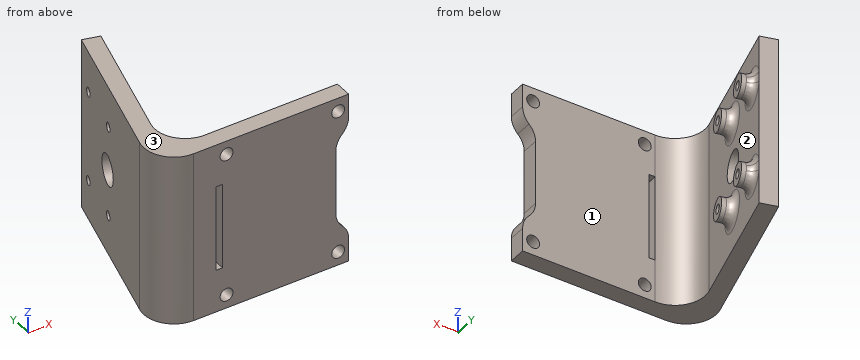
```python
from build123d import *
from build123d.topology import SkipClean

# Parameters (mm, degrees)
ESTRUSIONE_ESTRUSIONE1_DEPTH = 40
RACCORDO1_R                  = 7
SCHIZZO2_W                   = 1.5
SCHIZZO2_H                   = 20
TAGLIO_ESTRUSIONE1_DEPTH     = 40
SCHIZZO3_R                   = 1.05
SCHIZZO3_R_2                 = 3.5
TAGLIO_ESTRUSIONE2_DEPTH     = 40
SCHIZZO4_R                   = 2.5
SCHIZZO4_R_2                 = 1.05
ESTRUSIONE_ESTRUSIONE2_DEPTH = 3
RACCORDO2_R                  = 2
SCHIZZO5_R                   = 1.5
TAGLIO_ESTRUSIONE3_DEPTH     = 17
TAGLIO_ESTRUSIONE4_DEPTH     = 10
RACCORDO3_R                  = 5
RACCORDO4_R                  = 5


with BuildPart() as part:
    # Schizzo1 → Estrusione-Estrusione1 (new body)
    with BuildSketch(Plane.XY):
        Polygon((0, 0), (-40, 0), (-29.647238196, 38.637033052), (-33.510941501, 39.672309232), (-45.212901491, -4), (0, -4), align=None)
    extrude(amount=ESTRUSIONE_ESTRUSIONE1_DEPTH)

    # Raccordo1
    raccordo1_edges = [part.edges().sort_by_distance(p)[0] for p in [
        (-45.212901491, -4, 20),
        (-40, 0, 20),
    ]]
    fillet(raccordo1_edges, radius=RACCORDO1_R)

    # Schizzo2 → Taglio-Estrusione1 (cut)
    with BuildSketch(Plane(origin=(0, 0, 0), x_dir=(1, 0, 0), z_dir=(0, 1, 0))):
        with Locations((-30.12742239, -20)):
            Rectangle(SCHIZZO2_W, SCHIZZO2_H)
    extrude(amount=-TAGLIO_ESTRUSIONE1_DEPTH, mode=Mode.SUBTRACT)

    # Schizzo3 → Taglio-Estrusione2 (cut)
    with BuildSketch(Plane(origin=(-41.184211381, 11.03527618, 0), x_dir=(0, 0, 1), z_dir=(-0.9659258262890673, 0.2588190451025247, 0))):
        with Locations(Location((30.402866557, 25.309568218, 0), (0, 0, 270))):
            Circle(SCHIZZO3_R)
        with Locations(Location((9.20859967, 25.309568218, 0), (0, 0, 270))):
            Circle(SCHIZZO3_R)
        with Locations(Location((30.402866557, 13.009568218, 0), (0, 0, 270))):
            Circle(SCHIZZO3_R)
        with Locations(Location((9.20859967, 13.009568218, 0), (0, 0, 270))):
            Circle(SCHIZZO3_R)
        with Locations(Location((19.902866557, 13.409568216, 0), (0, 0, 270))):
            Circle(SCHIZZO3_R_2)
    extrude(amount=-TAGLIO_ESTRUSIONE2_DEPTH, mode=Mode.SUBTRACT)

    # Schizzo4 → Estrusione-Estrusione2 (add)
    # profile 1 of 4: a face of its own
    with SkipClean():  # the faces are left unmerged after this step: merging them gives an invalid solid
        with BuildSketch(Plane(origin=(-37.320508076, 10, 0), x_dir=(0, 0, -1), z_dir=(0.9659258262890674, -0.2588190451025245, 0))):
            with Locations(Location((-9.20859967, 13.009568218, 0), (0, 0, 270))):
                Circle(SCHIZZO4_R)
            with Locations(Location((-9.20859967, 13.009568218, 0), (0, 0, 90))):
                Circle(SCHIZZO4_R_2, mode=Mode.SUBTRACT)
        # profile 2 of 4: a face of its own
        with BuildSketch(Plane(origin=(-37.320508076, 10, 0), x_dir=(0, 0, -1), z_dir=(0.9659258262890674, -0.2588190451025245, 0))):
            with Locations(Location((-30.402866557, 13.009568218, 0), (0, 0, 270))):
                Circle(SCHIZZO4_R)
            with Locations(Location((-30.402866557, 13.009568218, 0), (0, 0, 270))):
                Circle(SCHIZZO4_R_2, mode=Mode.SUBTRACT)
        # profile 3 of 4: a face of its own
        with BuildSketch(Plane(origin=(-37.320508076, 10, 0), x_dir=(0, 0, -1), z_dir=(0.9659258262890674, -0.2588190451025245, 0))):
            with Locations(Location((-30.402866557, 25.309568218, 0), (0, 0, 270))):
                Circle(SCHIZZO4_R)
            with Locations(Location((-30.402866557, 25.309568218, 0), (0, 0, 270))):
                Circle(SCHIZZO4_R_2, mode=Mode.SUBTRACT)
        # profile 4 of 4: a face of its own
        with BuildSketch(Plane(origin=(-37.320508076, 10, 0), x_dir=(0, 0, -1), z_dir=(0.9659258262890674, -0.2588190451025245, 0))):
            with Locations(Location((-9.20859967, 25.309568218, 0), (0, 0, 270))):
                Circle(SCHIZZO4_R)
            with Locations(Location((-9.20859967, 25.309568218, 0), (0, 0, 90))):
                Circle(SCHIZZO4_R_2, mode=Mode.SUBTRACT)
        extrude(amount=ESTRUSIONE_ESTRUSIONE2_DEPTH)
    add(part.part.scale(1), mode=Mode.REPLACE)  # the faces are merged on a copy

    # Raccordo2
    raccordo2_edges = [part.edges().sort_by_distance(p)[0] for p in [
        (-30.122862185, 36.86198016, 9.20859967),
        (-33.306336439, 24.981092497, 9.20859967),
        (-33.306336439, 24.981092497, 30.402866557),
        (-30.122862185, 36.86198016, 30.402866557),
    ]]
    fillet(raccordo2_edges, radius=RACCORDO2_R)

    # Schizzo5 → Taglio-Estrusione3 (cut)
    with BuildSketch(Plane(origin=(0, 0, 0), x_dir=(1, 0, 0), z_dir=(0, 1, 0))):
        with Locations(Location((-2.444220089, -36.8336475, 0), (0, 0, 180))):
            Circle(SCHIZZO5_R)
        with Locations(Location((-2.444220089, -3.1663525, 0), (0, 0, 180))):
            Circle(SCHIZZO5_R)
        with Locations(Location((-28.433202301, -3.1663525, 0), (0, 0, 180))):
            Circle(SCHIZZO5_R)
        with Locations(Location((-28.433202301, -36.8336475, 0), (0, 0, 180))):
            Circle(SCHIZZO5_R)
    extrude(amount=-TAGLIO_ESTRUSIONE3_DEPTH, mode=Mode.SUBTRACT)

    # Schizzo6 → Taglio-Estrusione4 (cut)
    with BuildSketch(Plane(origin=(0, 0, 0), x_dir=(1, 0, 0), z_dir=(0, 1, 0))):
        Polygon((0, -20), (0, -30), (-3, -30), (-3, -10), (0, -10), align=None)
    extrude(amount=-TAGLIO_ESTRUSIONE4_DEPTH, mode=Mode.SUBTRACT)

    # Raccordo3
    # the kernel refuses this fillet: 5 mm, written as the material it takes off along each edge
    with BuildSketch(Plane(origin=(0, 11.456439237, 10), x_dir=(0, 0, -1), z_dir=(0, -1, 0))) as raccordo3_piece_1:
        with BuildLine():
            CenterArc((4.582575695, -5), RACCORDO3_R, 90, 66.421821522)
            Line((0, -3), (-0.091651514, -2.96))
            ThreePointArc((-0.091651514, -2.96), (-0.1, -1.5), (-0.1, 0))
            Line((-0.1, 0), (0, 0.1))
            Line((0, 0.1), (4.582575695, 0.1))
            Line((4.582575695, 0.1), (4.582575695, 0))
        make_face()
    extrude(amount=26.912878475, mode=Mode.SUBTRACT)
    with BuildSketch(Plane(origin=(0, 11.456439237, 30), x_dir=(0, 0, 1), z_dir=(0, -1, 0))) as raccordo3_piece_2:
        with BuildLine():
            CenterArc((4.582575695, 5), RACCORDO3_R, 203.578178478, 66.421821522)
            Line((0, 3), (-0.091651514, 2.96))
            ThreePointArc((-0.091651514, 2.96), (-0.1, 1.5), (-0.1, 0))
            Line((-0.1, 0), (0, -0.1))
            Line((0, -0.1), (4.582575695, -0.1))
            Line((4.582575695, -0.1), (4.582575695, 0))
        make_face()
    extrude(amount=26.912878475, mode=Mode.SUBTRACT)

    # Raccordo4
    raccordo4_edges = [part.edges().sort_by_distance(p)[0] for p in [
        (-3, -2, 30),
        (-3, -2, 10),
    ]]
    fillet(raccordo4_edges, radius=RACCORDO4_R)


solid = part.part
```
Check sheet for the modelled part. Datum: model origin and axes. Units: mm. Face numbers are marked on the shaded views. Give positions to 0.01 mm unless a question says otherwise; leave off trailing zeros. Loops run counter-clockwise (first coordinate to the right, second up) from the corner with the lowest first, then second, coordinate; pieces in that order, holes last. Notation, with made-up numbers: M -26.5,8 L -6.5,8 A35 cw -6.5,46 Z; hole C -17.75,16 d8. An arc over 180 degrees is marked long. Answer as CSV lines item,"result".
Item 1: Draft check along Z on the marked faces 1, 2 and 3. Enter one of: pulls with the +Z half, pulls with the -Z half, needs draft (parallel to the pull), parting line crosses it, or undercut.
Reply:
face 1,"needs draft"
face 2,"undercut"
face 3,"pulls with the +Z half"
Item 2: Scan lines: L1, parallel to X at y = -0.5, z = 36; L2, parallel to Y at x = -26, z = 20; L3, parallel to X at y = 21.5, z = 38.5. Record each from-to range of solid material in increasing order.
Reply:
L1,"-42.15 to -29.68, -27.19 to -3.69, -1.2 to 0"
L2,"-4 to 0"
L3,"-38.38 to -34.24"
Item 3: Sectioned sample at C-C, the plane y = 7.5. Enter the section's corners in (x, z).
Reply:
outline,"M -42.13,0 L -37.86,0 L -37.86,40 L -42.13,40 Z"
Item 4: Depth check by flat-ended pin: pin 1 Ø6 at (x, z) = (-4.5, 5) entering from +Y; pin 2 Ø1.5 at (y, z) = (31, 35.5) entering from -X; pin 3 Ø2 at (y, z) = (-1.5, 25) entering from -X. Enter the tip coordinate at first touch or a pass-through.
Reply:
pin 1,"y = 0"
pin 2,"x = -36.04"
pin 3,"x = -42.15"
Item 5: Sectioned sample at A-A, the plane z = 36. Enter the section's corners in (x, y).
Reply:
outline,"M -42.85,4.81 A7 ccw -36.09,-4 L -29.68,-4 L -29.68,0 L -30.88,0 A7 cw -37.64,8.81 L -29.65,38.64 L -33.51,39.67 Z; M -27.19,-4 L -3.69,-4 L -3.69,0 L -27.19,0 Z; M -1.2,-4 L 0,-4 L 0,0 L -1.2,0 Z"
Item 6: Sectioned sample at B-B, the plane x = -18.5. Enter the section's corners in (y, z), then the cut area to 3 significant figures.
Reply:
outline,"M -4,0 L 0,0 L 0,40 L -4,40 Z"
area,"160 mm^2"
